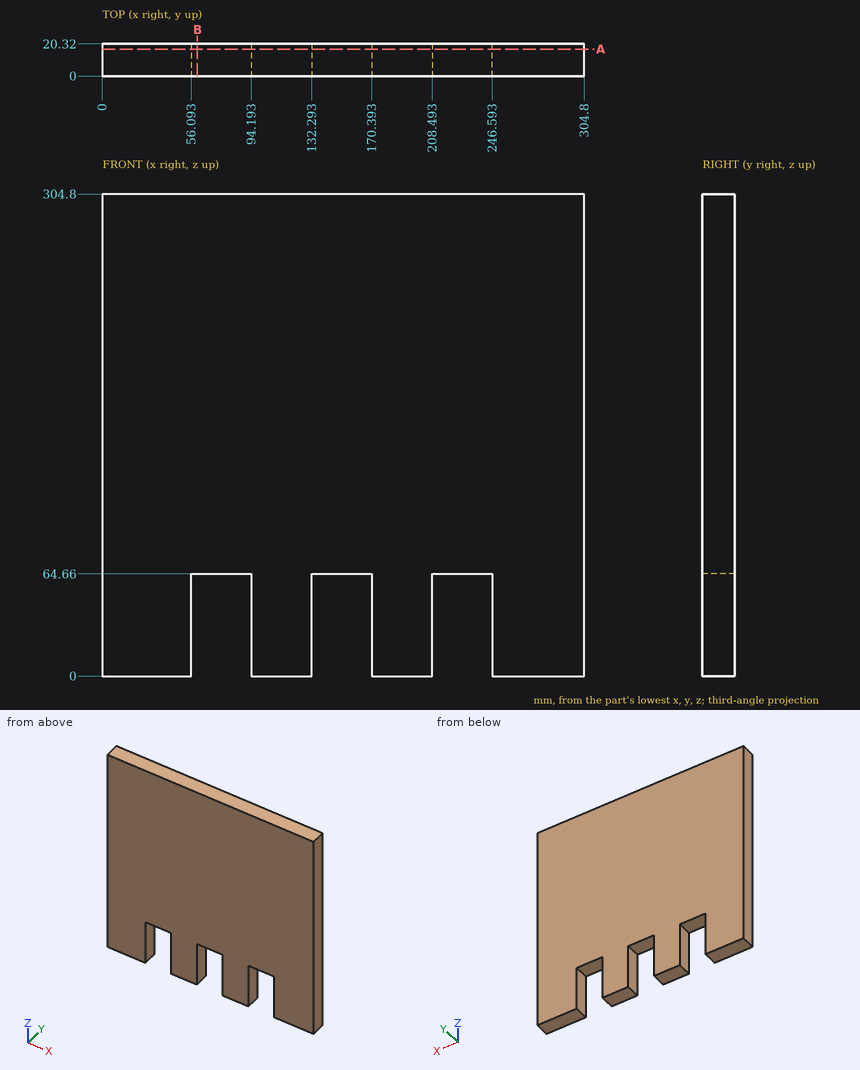
Input: dimensioned drawing with shaded views. Units: mm. Origin: part minimum x, y, z. Give positions to 0.01 mm unless a question says otherwise; leave off trailing zeros. Write each loop counter-clockwise with the first axis right and the second up, starting at its lowest first coordinate (ties: lowest second). Pieces come first, ordered by that corner, then holes. Notation, with made-up numbers: (68, 69.25) - (111, 69.25) arc R16 cw to (111, 76.25) - close; hole circle Ø3 at (70.5, -31.75). An arc over 180 degrees is marked (long way). Write item = value, one per line. Start each with the question number.
1) Cut plane A-A (y = 17). Return loops of the section in (x, z), and give its area (3 significant figures).
2) Material intervals for L1, parallel to X at y = 10.5, z = 23; L2, parallel to Z at x = 141.5, y = 7.25, sorted ascending. Write a range as [from, to].
3) Cut plane B-B (x = 60). Return loops of the section in (y, z).
4) Pin query (flat end, axial travel): pin 1 (5 mm diameter, centred on x = 150.5, y = 5, fed in from -Z). Return the tip coordinate at first contact, or that it passes through.
Answers follow:
q1.outline = (0, 0) - (56.09, 0) - (56.09, 64.66) - (94.19, 64.66) - (94.19, 0) - (132.29, 0) - (132.29, 64.66) - (170.39, 64.66) - (170.39, 0) - (208.49, 0) - (208.49, 64.66) - (246.59, 64.66) - (246.59, 0) - (304.8, 0) - (304.8, 304.8) - (0, 304.8) - close
q1.area = 85,500 mm^2
q2.L1 = [0, 56.09], [94.19, 132.29], [170.39, 208.49], [246.59, 304.8]
q2.L2 = [64.66, 304.8]
q3.outline = (0, 64.66) - (20.32, 64.66) - (20.32, 304.8) - (0, 304.8) - close
q4.pin_1 = 64.66
